Could you check a few things on this model? Use its own coordinates, in mm. A direction names the side the tool comes from. Give positions to 0.01 mm unless a question says otherwise; leave off trailing zeros. Order: outer loops, then holes, each group sorted by start corner. A loop starts at its lowest first (then second) coordinate and runs counter-clockwise, first axis right, second up.
from build123d import *

# Parameters (mm, degrees)
SKETCH1_R             = 7.223333333
BOSS_EXTRUDE1_DEPTH   = 52
BOSS_EXTRUDE1_2_DEPTH = 52
BOSS_EXTRUDE1_3_DEPTH = 52
BOSS_EXTRUDE1_4_DEPTH = 52
BOSS_EXTRUDE1_5_DEPTH = 52
BOSS_EXTRUDE1_6_DEPTH = 52
SKETCH2_W             = 43.346666666
SKETCH2_H             = 28.896666666
BOSS_EXTRUDE2_DEPTH   = 2
SKETCH3_W             = 43.346666666
SKETCH3_H             = 28.896666666
BOSS_EXTRUDE3_DEPTH   = 2
FILLET1_R             = 7.22


with BuildPart() as part:
    # Sketch1 → Boss-Extrude1 (new body)
    with BuildSketch(Plane(origin=(0, 0, 0), x_dir=(1, 0, 0), z_dir=(0, 1, 0))):
        with Locations(Location((0, 0, 0), (0, 0, 90))):
            Circle(SKETCH1_R)
    extrude(amount=BOSS_EXTRUDE1_DEPTH)



with BuildPart() as body_2:
    # Sketch1 → Boss-Extrude1 2 (new body)
    with BuildSketch(Plane(origin=(0, 0, 0), x_dir=(1, 0, 0), z_dir=(0, 1, 0))):
        with Locations(Location((14.45, 0, 0), (0, 0, 90))):
            Circle(SKETCH1_R)
    extrude(amount=BOSS_EXTRUDE1_2_DEPTH)


with BuildPart() as body_3:
    # Sketch1 → Boss-Extrude1 3 (new body)
    with BuildSketch(Plane(origin=(0, 0, 0), x_dir=(1, 0, 0), z_dir=(0, 1, 0))):
        with Locations(Location((28.9, 0, 0), (0, 0, 90))):
            Circle(SKETCH1_R)
    extrude(amount=BOSS_EXTRUDE1_3_DEPTH)


with BuildPart() as body_4:
    # Sketch1 → Boss-Extrude1 4 (new body)
    with BuildSketch(Plane(origin=(0, 0, 0), x_dir=(1, 0, 0), z_dir=(0, 1, 0))):
        with Locations(Location((14.45, 14.45, 0), (0, 0, 90))):
            Circle(SKETCH1_R)
    extrude(amount=BOSS_EXTRUDE1_4_DEPTH)


with BuildPart() as body_5:
    # Sketch1 → Boss-Extrude1 5 (new body)
    with BuildSketch(Plane(origin=(0, 0, 0), x_dir=(1, 0, 0), z_dir=(0, 1, 0))):
        with Locations(Location((28.9, 14.45, 0), (0, 0, 90))):
            Circle(SKETCH1_R)
    extrude(amount=BOSS_EXTRUDE1_5_DEPTH)


with BuildPart() as body_6:
    # Sketch1 → Boss-Extrude1 6 (new body)
    with BuildSketch(Plane(origin=(0, 0, 0), x_dir=(1, 0, 0), z_dir=(0, 1, 0))):
        with Locations(Location((0, 14.45, 0), (0, 0, 90))):
            Circle(SKETCH1_R)
    extrude(amount=BOSS_EXTRUDE1_6_DEPTH)


with BuildPart() as part_1:
    add(part.part)

    add(body_2.part)  # Boss-Extrude2 merges body 2

    add(body_3.part)  # Boss-Extrude2 merges body 3

    add(body_4.part)  # Boss-Extrude2 merges body 4

    add(body_5.part)  # Boss-Extrude2 merges body 5

    add(body_6.part)  # Boss-Extrude2 merges body 6
    # Sketch2 → Boss-Extrude2 (add)
    with BuildSketch(Plane(origin=(0, 52, 0), x_dir=(1, 0, 0), z_dir=(0, 1, 0))):
        with Locations((14.45, 7.225)):
            Rectangle(SKETCH2_W, SKETCH2_H)
    extrude(amount=-BOSS_EXTRUDE2_DEPTH)

    # Sketch3 → Boss-Extrude3 (add)
    with BuildSketch(Plane.XZ):
        with Locations((14.45, -7.225)):
            Rectangle(SKETCH3_W, SKETCH3_H)
    extrude(amount=-BOSS_EXTRUDE3_DEPTH)

    # Fillet1
    fillet1_edges = [part_1.edges().sort_by_distance(p)[0] for p in [
        (36.123333333, 51, 7.223333333),
        (36.123333333, 1, 7.223333333),
        (-7.223333333, 51, 7.223333333),
        (-7.223333333, 1, 7.223333333),
        (-7.223333333, 51, -21.673333333),
        (36.123333333, 51, -21.673333333),
        (36.123333333, 1, -21.673333333),
        (-7.223333333, 1, -21.673333333),
    ]]
    fillet(fillet1_edges, radius=FILLET1_R)


solid = part_1.part
Item 1: Imagine slicing it at B-B on z = -18.75. Give the number of separate pieces and of enclosed holes in the cut face, then the cut area to 3 significant figures.
Findings:
separate pieces: 1
enclosed holes: 2
area: 1,830 mm2
Item 2: Please list where these lines run through material, in increasing order: line 1 along X through (y, z) = (40.5, -16); line 2 along X through (y, z) = (25.5, -17.25); line 3 along Z through (x, y) = (18.5, 16.5).
Findings:
line 1: x = -7.06 to 7.06, 7.39 to 21.51, 21.84 to 35.96
line 2: x = -6.66 to 6.66, 7.79 to 21.11, 22.24 to 35.56
line 3: z = -20.43 to -8.47, -5.98 to 5.98
Item 3: Imagine slicing it at A-A on y = 33. List the corners of the cut face in (x, z) for me, then the cut area to 3 significant figures.
Findings:
outline: circle Ø14.45 at (0, -14.45); circle Ø14.45 at (0, 0); circle Ø14.45 at (14.45, -14.45); circle Ø14.45 at (14.45, 0); circle Ø14.45 at (28.9, -14.45); circle Ø14.45 at (28.9, 0)
area: 984 mm2
Item 4: For faces 1 (the cylindrical face through (-5.164, 1.014, -19.502)), 2 (the cylindrical face through (22.809, 25.664, -3.883)), which set-ups out of +Z, -Z, +X, -X, +Y, -Y let a thin tool reach every point of the face, with its end or its side?
Findings:
face 1: -Z, -X, +Y, -Y
face 2: none
Item 5: We'd pull the mould along Z, two halves only. Please class faces 3 (the flat face through (14, 51, -21.673)), 4 (the flat face through (11, 50, -7)), 5 (the flat face through (-7.223, 51, -7)): +Z half, -Z half, draft (parallel to the pull), parting line (faces both ways), or undercut.
Findings:
face 3: -Z half
face 4: undercut
face 5: draft
Item 6: Imagine slicing it at D-D on z = -6.25. List the corners of the cut face in (x, y) for me.
Findings:
outline: (-7.22, 0) - (36.12, 0) - (36.12, 2) - (32.52, 2) - (32.52, 50) - (36.12, 50) - (36.12, 52) - (-7.22, 52) - (-7.22, 50) - (-3.62, 50) - (-3.62, 2) - (-7.22, 2) - close; hole (3.62, 2) - (10.83, 2) - (10.83, 50) - (3.62, 50) - close; hole (18.07, 2) - (25.28, 2) - (25.28, 50) - (18.07, 50) - close
Item 7: For pin 1 (1 mm diameter, centred on x = 21.5, y = 28, fed in from +Z); pin 2 (10 mm diameter, centred on x = 23, y = 18.5, fed in from +Z); pin 3 (1.5 mm diameter, centred on x = 8.5, y = 34.5, fed in from +Z), each with a flat end and sliding along its axis, tell me the tip position at first contact or that it passes through.
Findings:
pin 1: stops at z = 3.05
pin 2: stops at z = 7.17
pin 3: stops at z = 5.01
Item 8: Imagine slicing it at C-C on x = 8. List the corners of the cut face in (y, z) for me.
Findings:
outline: (0, -21.67) - (2, -21.67) - (2, -17.7) - (50, -17.7) - (50, -21.67) - (52, -21.67) - (52, 7.22) - (50, 7.22) - (50, 3.25) - (2, 3.25) - (2, 7.22) - (0, 7.22) - close; hole (2, -11.2) - (50, -11.2) - (50, -3.25) - (2, -3.25) - close
